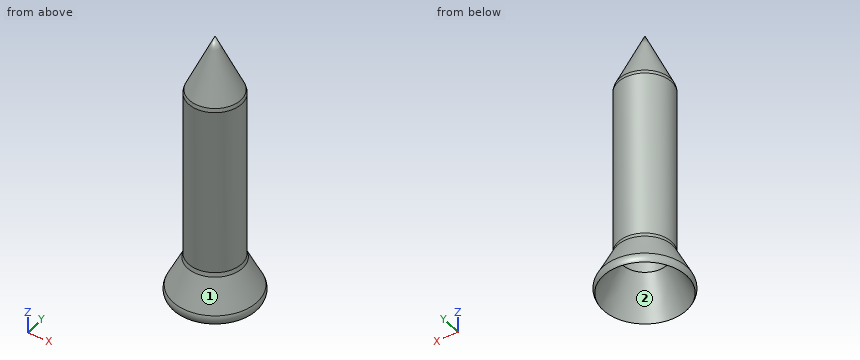
from build123d import *

# Parameters (mm, degrees)
F3_T = -2.54
F4_R = 5.08


# Not quite as in the source:
# - a fillet or chamfer that OpenCascade refuses, or shapes differently, is made with other operations: its cross-section is extruded or revolved along the edge and cut away or added


with BuildPart() as f2:
    # F0 (on Right) → F2 (revolve)
    with BuildSketch(Plane.YZ):
        Polygon((0, -77.1136805415), (0, 0), (0, 75.9008899331), (-15.0823583826, 43.1482791901), (-15.0823583826, -54.3898443918), (-26.3941269368, -77.1136805415), align=None)
    revolve(axis=Axis((0, 0, 37.9504449666), (0, 0, 1)))

    # F3
    f3_openings = [f2.faces().sort_by_distance(p)[0] for p in [
        (0, 0, -77.113681),
    ]]
    offset(amount=F3_T, openings=f3_openings, kind=Kind.INTERSECTION)

    # F4
    f4_edges = [f2.edges().sort_by_distance(p)[0] for p in [
        (0, 15.082358, 43.148279),
        (0, 15.082358, -54.389844),
        (0, -15.082358, -5.620783),
    ]]
    fillet(f4_edges, radius=F4_R)

    # F5: fillet of radius 5.08 on 3 edges, made by hand

    # F5_s1 → F5_t2 (revolve, cut)
    with BuildSketch(Plane.YZ):
        with BuildLine():
            ThreePointArc((-23.8701527835, -72.0433526939), (-24.3927830464, -74.6204948412), (-23.5568230573, -77.1136805415))
            Line((-23.5568230573, -77.1136805415), (-26.3941269368, -77.1136805415))
            Line((-26.3941269368, -77.1136805415), (-23.8701527835, -72.0433526939))
        make_face()
    revolve(axis=Axis((0, 0, -77.1136805415), (0, 0, 1)), mode=Mode.SUBTRACT)


solid = f2.part
Input: part model. Units: mm. Frame: model coordinates. Face numbers are marked on the shaded views. Coordinates: 2 decimals unless noted, no trailing zeros. Order: outer loops, then holes, each group sorted by start corner. A loop starts at its lowest first (then second) coordinate and runs counter-clockwise, first axis right, second up. Notation, with made-up numbers: M -30.5,-36 L 10.5,-36 A14 ccw 10.5,-13 Z; hole C 44.25,68.5 d9. An arc over 180 degrees is marked long. Answer in a Markdown table with one row per item.
(1) Section query B-B, the plane z = 62. Output: boundary loops of the cut face in (x, y).
Numbers:
| item | result |
|---|---|
| outline | C 0,0 d12.8; hole C 0,0 d7.21 |
(2) Section query A-A, the plane z = 22. Output: boundary loops of the cut face in (x, y).
Numbers:
| item | result |
|---|---|
| outline | C 0,0 d30.16; hole C 0,0 d25.08 |
(3) Material intervals for line 1 (X direction, y = 0, z = 12.5); line 2 (X direction, y = 4, z = -58); line 3 (Y direction, x = 3, z = -40), sorted ascending. Write a range as [from, to].
Numbers:
| item | result |
|---|---|
| line 1 | x = [-15.08, -12.54], [12.54, 15.08] |
| line 2 | x = [-16.4, -13.46], [13.46, 16.4] |
| line 3 | y = [-14.78, -12.18], [12.18, 14.78] |
(4) Draft query along Y for the marked faces 1 and 2. Return one class per face: pulls with the +Y half, pulls with the -Y half, needs draft (parallel to the pull), parting line crosses it, or undercut.
Numbers:
| item | result |
|---|---|
| face 1 | parting line crosses it |
| face 2 | undercut |
(5) Contact query for flat-ended pins moving along their axis: pin 1 Ø1.5 at (x, z) = (-8.5, 46) entering from -Y; pin 2 Ø22.5 at (x, y) = (0, 0) entering from -Z; pin 3 Ø6 at (x, y) = (4.5, 3.5) entering from +Z. Output: stop coordinate, or through.
Numbers:
| item | result |
|---|---|
| pin 1 | stops at y = -11.53 |
| pin 2 | stops at z = 45.4 |
| pin 3 | stops at z = 70.04 |
